Geometry check sheet. Reference: the model listing, model coordinates, mm. A direction names the side the tool comes from. Round coordinates to 2 decimals unless told otherwise and drop trailing zeros. Loops run counter-clockwise (first coordinate to the right, second up) from the corner with the lowest first, then second, coordinate; pieces in that order, holes last. Notation, with made-up numbers: (36.5, -18) -> (51.5, -18) arc R20 ccw to (51.5, 7) -> close; hole circle Ø1 at (51, 43). An arc over 180 degrees is marked (long way). Use one line per item in the form item = value.
from build123d import *

# Parameters (mm, degrees)
SKETCH_1_W      = 60
SKETCH_1_H      = 50
EXTRUDE_1_DEPTH = 10
SKETCH_8_W      = 60
SKETCH_8_H      = 60
EXTRUDE_2_DEPTH = 10
SKETCH_9_R      = 4.75
SKETCH_9_R_2    = 4.25
EXTRUDE_3_DEPTH = 10
FILLET_1_RADIUS = 30
FILLET_1_LENGTH = 10
CHAMFER_1_SIZE  = 1
HOLE_WIZARD_4_D = 3.2


with BuildPart() as part:
    # 草图1 → 凸台-拉伸1 (new body)
    with BuildSketch(Plane.XY):
        Rectangle(SKETCH_1_W, SKETCH_1_H)
    extrude(amount=EXTRUDE_1_DEPTH)

    # 草图3 → 孔1 (revolve, cut)
    with BuildSketch(Plane(origin=(0, 0, 10), x_dir=(0, -1, 0), z_dir=(1, 0, 0))):
        Polygon((0, 0), (0, 10), (4, 10), (4, 0.603553391), (4.25, 0), align=None)
    revolve(axis=Axis((0, 0, 16.445314094), (0, 0, -1)), mode=Mode.SUBTRACT)

    # 草图8 → 凸台-拉伸2 (add)
    with BuildSketch(Plane.XZ.offset(25)):
        with Locations((0, 5)):
            Rectangle(SKETCH_8_W, SKETCH_8_H)
    extrude(amount=EXTRUDE_2_DEPTH)

    # 草图9 → 凸台-拉伸3 (add)
    with BuildSketch(Plane.XY.offset(10)):
        with Locations(Location((0, 0, 0), (0, 0, 180))):
            Circle(SKETCH_9_R)
        Circle(SKETCH_9_R_2, mode=Mode.SUBTRACT)
    extrude(amount=EXTRUDE_3_DEPTH)

    # 圆角1: full round fillet: the end face becomes a half cylinder, R = half its width
    fillet_1_face = Plane((0, 25, 5), x_dir=(0, 0, 1), z_dir=(0, 1, 0))  # on the end face: x along it, z out of the body
    fillet_1_slab = fillet_1_face.offset(-FILLET_1_RADIUS / 2) * Box(FILLET_1_LENGTH, 2 * FILLET_1_RADIUS, FILLET_1_RADIUS, mode=Mode.PRIVATE)  # the body's end, R deep
    fillet_1_round = Plane((0, -5, 5), x_dir=(0, 1, 0), z_dir=(0, 0, 1)) * Cylinder(FILLET_1_RADIUS, FILLET_1_LENGTH, mode=Mode.PRIVATE)  # its axis R under the face
    add(fillet_1_slab - fillet_1_round, mode=Mode.SUBTRACT)

    # 倒角1
    chamfer_1_edges = [part.edges().sort_by_distance(p)[0] for p in [
        (30, -25, -12.5),
        (30, -25, 22.5),
        (30, -30, -25),
        (0, -25, 35),
        (30, -30, 35),
        (-30, -25, 22.5),
        (-30, -25, -12.5),
        (-30, -30, 35),
        (0, -25, -25),
        (-30, -30, -25),
        (30, -35, 5),
        (0, -35, 35),
        (-30, -35, 5),
        (0, -35, -25),
        (-30, -15, 0),
        (-30, -15, 10),
        (0, 25, 10),
        (0, 25, 0),
        (30, -15, 10),
        (30, -15, 0),
    ]]
    chamfer(chamfer_1_edges, length=CHAMFER_1_SIZE)

    # 孔4 (through all)
    with Locations(Plane(origin=(0, -25, 0), x_dir=(1, 0, 0), z_dir=(0, 1, 0))):
        with Locations((-19, 14), (19, 14), (19, -24), (-19, -24)):
            Hole(HOLE_WIZARD_4_D / 2)


solid = part.part
1. Material ranges on line 1 along X through (y, z) = (-27.75, 24); line 2 along Z through (x, y) = (19, -32.75); line 3 along X through (y, z) = (0, 4.25), recorded low to high.
Return value:
line_1 = -30 to -20.6, -17.4 to 17.4, 20.6 to 30
line_2 = -25 to -15.6, -12.4 to 22.4, 25.6 to 35
line_3 = -29.58 to -4, 4 to 29.58
2. Section check A-A (z = -14). Record the boundary of the cut face in (x, y), then the cut area to 3 significant figures.
Return value:
outline = (-30, -34) -> (-29, -35) -> (-20.6, -35) -> (-20.6, -25) -> (-29, -25) -> (-30, -26) -> close; (-17.4, -35) -> (17.4, -35) -> (17.4, -25) -> (-17.4, -25) -> close; (20.6, -35) -> (29, -35) -> (30, -34) -> (30, -26) -> (29, -25) -> (20.6, -25) -> close
area = 534 mm2
3. Section check D-D (z = 27). Record the boundary of the cut face in (x, y).
Return value:
outline = (-30, -34) -> (-29, -35) -> (29, -35) -> (30, -34) -> (30, -26) -> (29, -25) -> (-29, -25) -> (-30, -26) -> close
4. Gauge pin test, flat ends, axial feed: pin 1 (7.5 mm diameter, centred on x = -2, y = -2, fed in from +Z); pin 2 (4 mm diameter, centred on x = -19, z = -14, fed in from +Y); pin 3 (8 mm diameter, centred on x = -17.5, y = 15, fed in from +Z). Record the tip position at first contact, or that the pin passes through.
Return value:
pin_1 = 20
pin_2 = -25
pin_3 = 10
5. Section check C-C (y = -24). Record the boundary of the cut face in (x, z).
Return value:
outline = (-30, 1) -> (-29, 0) -> (29, 0) -> (30, 1) -> (30, 9) -> (29, 10) -> (-29, 10) -> (-30, 9) -> close
6. Section check B-B (x = 0). Record the boundary of the cut face in (y, z), then the cut area to 3 significant figures.
Return value:
outline = (-35, -24) -> (-34, -25) -> (-26, -25) -> (-25, -24) -> (-25, 0) -> (-4, 0) -> (-4, 9.4) -> (-4.25, 10) -> (-4.25, 20) -> (-4.75, 20) -> (-4.75, 10) -> (-25, 10) -> (-25, 34) -> (-26, 35) -> (-34, 35) -> (-35, 34) -> close; (4, 0) -> (24, 0) -> (25, 1) -> (25, 9) -> (24, 10) -> (4.75, 10) -> (4.75, 20) -> (4.25, 20) -> (4.25, 10) -> (4, 9.4) -> close
area = 1,030 mm2
7. Mould release check, pull along Y, two halves, no side actions. Record for faces 1 (the cylindrical face through (1.03, 4.637, 14.93)), 2 (the cylindrical face through (0.66, 24.993, 5.056)), 3 (the flat face through (0, -35, 5)), 4 (the cylindrical face through (-17.82, -30.07, -15.08)): released by +Y, released by -Y, zero draft, split by the parting line, or undercut.
Return value:
face_1 = undercut
face_2 = released by +Y
face_3 = released by -Y
face_4 = zero draft
8. Tool access check on faces 5 (the cylindrical face through (2.285, 3.584, 14.93)), 6 (the flat face through (4, 2, 20)), 7 (the flat face through (0, -25, -12)). Record the directions out of +Z, -Z, +X, -X, +Y, -Y that give a thin tool (end or side, any length) a straight path to the whole face; none if there is none.
Return value:
face_5 = +Z
face_6 = +Z, +X, -X, +Y
face_7 = -Z, +X, -X, +Y
